Geometry check sheet. Reference: the model listing, model coordinates, mm. A direction names the side the tool comes from. Give positions to 0.01 mm unless a question says otherwise; leave off trailing zeros. Order: outer loops, then holes, each group sorted by start corner. A loop starts at its lowest first (then second) coordinate and runs counter-clockwise, first axis right, second up. Notation, with made-up numbers: M 24.5,-26.5 L 69.5,-26.5 A19 ccw 69.5,-10.5 Z; hole C 37,81.25 d9. An arc over 180 degrees is marked long. Put each result on its own line as item: value. Start each with the question number.
Q1. Section check A-A on x = 25. Record the cut outline in (y, z).
Q2. Mould release check, pull along Z, two halves, no side actions. Record for faces 4 (the cylindrical face through (30.534, 0.507, 13.236)), 5 (the cylindrical face through (55.5, 24.9, 13)), 6 (the flat face through (56, 18, 16)), 7 (the flat face through (0.5, 34, 31)): +Z half, -Z half, draft (parallel to the pull), parting line (faces both ways), or undercut.
Q3. Section check B-B on z = 21.5. Record the cut outline in (x, y), then the cut area to 3 significant figures.
Q4. Section check C-C on y = 3.5. Record the cut outline in (x, z), then the cut area to 3 significant figures.
Q5. Section check D-D on y = 25. Record the cut outline in (x, z).
Q6. Access from +Z, -Z, +X, -X, +Y, -Y to the whole of each face (thin tool, end or side, straight path). Record for faces 1 (the cylindrical face through (55.4, 0.57, 15.78)), 2 (the flat face through (1, 18, 16)), 3 (the cylindrical face through (55.507, 25.22, 27.496)).
Q7. Material ranges on L1, parallel to X at y = 13.5, z = 7; L2, parallel to Y at x = 23, z = 21, recorded low to high.
Q8. Go/stop test with flat-tipped pins: pin 1 (15.5 mm diameter, centred on y = 25, z = 21.5, fed in from +X); pin 2 (3 mm diameter, centred on x = 37.5, z = 3.5, fed in from +Y). Record where each tip stops, or that it passes through.
```python
from build123d import *

# Parameters (mm, degrees)
BASE_FLANGE1_DEPTH = 32
CUT_EXTRUDE1_DEPTH = 10
SKETCH9_R          = 4
CUT_EXTRUDE2_DEPTH = 10
SKETCH10_R         = 3.75
CUT_EXTRUDE3_DEPTH = 10
CHAMFER2_SIZE      = 2


# Sheet-metal steps are written as plain solids
with BuildPart() as part:
    # Sketch1 → Base-Flange1 (new body)
    with BuildSketch(Plane.XY):
        with BuildLine():
            Line((0, 35), (0, 2))
            ThreePointArc((0, 2), (0.585786438, 0.585786438), (2, 0))
            Line((2, 0), (54, 0))
            ThreePointArc((54, 0), (55.414213562, 0.585786438), (56, 2))
            Line((56, 2), (56, 35))
            Line((56, 35), (55, 35))
            Line((55, 35), (55, 2))
            ThreePointArc((55, 2), (54.707106781, 1.292893219), (54, 1))
            Line((54, 1), (2, 1))
            ThreePointArc((2, 1), (1.292893219, 1.292893219), (1, 2))
            Line((1, 2), (1, 35))
            Line((1, 35), (0, 35))
        make_face()
    extrude(amount=BASE_FLANGE1_DEPTH)

    # Sketch8 → Cut-Extrude1 (cut)
    with BuildSketch(Plane(origin=(56, 0, 0), x_dir=(0, 0, -1), z_dir=(1, 0, 0))):
        with BuildLine():
            ThreePointArc((-16.295454545, 27.985415651), (-27.5, 25), (-16.295454545, 22.014584349))
            ThreePointArc((-16.295454545, 22.014584349), (-13, 25), (-16.295454545, 27.985415651))
        make_face()
    extrude(amount=-CUT_EXTRUDE1_DEPTH, mode=Mode.SUBTRACT)

    # Sketch9 → Cut-Extrude2 (cut)
    with BuildSketch(Plane.ZY):
        with Locations((21.5, 25)):
            Circle(SKETCH9_R)
    extrude(amount=-CUT_EXTRUDE2_DEPTH, mode=Mode.SUBTRACT)

    # Sketch10 → Cut-Extrude3 (cut)
    with BuildSketch(Plane(origin=(0, 1, 0), x_dir=(1, 0, 0), z_dir=(0, 1, 0))):
        with Locations(Location((28, -16, 0), (0, 0, 270))):
            Circle(SKETCH10_R)
    extrude(amount=-CUT_EXTRUDE3_DEPTH, mode=Mode.SUBTRACT)

    # Chamfer2
    chamfer2_edges = [part.edges().sort_by_distance(p)[0] for p in [
        (0.5, 35, 0),
        (55.5, 35, 0),
        (0.5, 35, 32),
        (55.5, 35, 32),
    ]]
    chamfer(chamfer2_edges, length=CHAMFER2_SIZE)


solid = part.part
```
Results found:
1. outline: M 0,0 L 1,0 L 1,13.75 L 0,13.75 Z; M 0,18.25 L 1,18.25 L 1,32 L 0,32 Z
2. face 4: undercut
2. face 5: undercut
2. face 6: draft
2. face 7: +Z half
3. outline: M 0,2 A2 ccw 2,0 L 54,0 A2 ccw 56,2 L 56,19 L 55,19 L 55,2 A1 cw 54,1 L 2,1 A1 cw 1,2 L 1,21 L 0,21 Z; M 0,29 L 1,29 L 1,35 L 0,35 Z; M 55,31 L 56,31 L 56,35 L 55,35 Z
3. area: 103 mm^2
4. outline: M 0,0 L 1,0 L 1,32 L 0,32 Z; M 55,0 L 56,0 L 56,32 L 55,32 Z
4. area: 64.0 mm^2
5. outline: M 0,0 L 1,0 L 1,17.5 L 0,17.5 Z; M 0,25.5 L 1,25.5 L 1,32 L 0,32 Z; M 55,0 L 56,0 L 56,13 L 55,13 Z; M 55,27.5 L 56,27.5 L 56,32 L 55,32 Z
6. face 1: +Z, -Z, +X, -Y
6. face 2: +Z, -Z, +Y
6. face 3: +X
7. L1: x = 0 to 1, 55 to 56
7. L2: y = 0 to 1
8. pin 1: stops at x = 56
8. pin 2: stops at y = 1
